```python
from build123d import *
from build123d.topology import SkipClean

# Parameters (mm, degrees)
SKETCH_1_R               = 22.5
EXTRUDE_1_DEPTH          = 13.4
SKETCH_2_R               = 2.1
EXTRUDE_2_DEPTH          = 4
FILLET_1_R               = 3.69
EXTRUDE_3_DEPTH          = 9.5
EXTRUDE_5_DEPTH          = 2
EXTRUDE_4_DEPTH          = 4.5
CUT_EXTRUDE_START        = -11
SKETCH_5_R               = 21.001588026
CUT_EXTRUDE_1_DEPTH      = 11
SKETCH_6_R               = 8
CUT_EXTRUDE_2_DEPTH      = 3
PATTERN_CIRCULAR_1_COUNT = 3
EXTRUDE_START            = -9
EXTRUDE_6_DEPTH          = 9
EXTRUDE_7_DEPTH          = 1
EXTRUDE_8_DEPTH          = 7
CHAMFER_1_SIZE           = 0.5
SKETCH_13_R              = 9.5
CUT_EXTRUDE_4_DEPTH      = 2
EXTRUDE_10_DEPTH         = 13.4


with BuildPart() as part:
    # Эскиз1 → Бобышка-Вытянуть1 (new body)
    with BuildSketch(Plane(origin=(0, 0, 0), x_dir=(1, 0, 0), z_dir=(0, 1, 0))):
        with Locations(Location((0, 0, 0), (0, 0, 270))):
            Circle(SKETCH_1_R)
    extrude(amount=EXTRUDE_1_DEPTH)

    # Эскиз2 → Бобышка-Вытянуть2 (add)
    # profile 1 of 2: a face of its own
    with BuildSketch(Plane.XZ):
        with BuildLine():
            Line((22.193692798, 3.7), (32.5, 3.7))
            Line((32.5, 3.7), (32.5, -3.7))
            Line((32.5, -3.7), (22.193692798, -3.7))
            ThreePointArc((22.193692798, -3.7), (22.5, 0), (22.193692798, 3.7))
        make_face()
        with Locations(Location((28.5, 0, 0), (0, 0, 270))):
            Circle(SKETCH_2_R, mode=Mode.SUBTRACT)
    # profile 2 of 2: a face of its own
    with BuildSketch(Plane.XZ):
        with BuildLine():
            Line((-22.193692798, -3.7), (-32.5, -3.7))
            Line((-32.5, -3.7), (-32.5, 3.7))
            Line((-32.5, 3.7), (-22.193692798, 3.7))
            ThreePointArc((-22.193692798, 3.7), (-22.5, 0), (-22.193692798, -3.7))
        make_face()
        with Locations(Location((-28.5, 0, 0), (0, 0, 90))):
            Circle(SKETCH_2_R, mode=Mode.SUBTRACT)
    extrude(amount=-EXTRUDE_2_DEPTH)

    # Скругление1
    fillet_1_edges = [part.edges().sort_by_distance(p)[0] for p in [
        (-32.5, 2, -3.7),
        (-32.5, 2, 3.7),
        (32.5, 2, 3.7),
        (32.5, 2, -3.7),
    ]]
    fillet(fillet_1_edges, radius=FILLET_1_R)

    # Эскиз3 → Бобышка-Вытянуть3 (add)
    with BuildSketch(Plane(origin=(0, 13.4, 0), x_dir=(1, 0, 0), z_dir=(0, 1, 0))):
        with BuildLine():
            Line((-1, 22.477766793), (-1, 20.977766793))
            ThreePointArc((-1, 20.977766793), (0, 21.001588026), (1, 20.977766793))
            Line((1, 20.977766793), (1, 22.477766793))
            ThreePointArc((1, 22.477766793), (0, 22.5), (-1, 22.477766793))
        make_face()
        with BuildLine():
            Line((19.966317063, -10.372857993), (18.667278957, -9.622857993))
            ThreePointArc((18.667278957, -9.622857993), (18.18790875, -10.500794013), (17.667278957, -11.3549088))
            Line((17.667278957, -11.3549088), (18.966317063, -12.1049088))
            ThreePointArc((18.966317063, -12.1049088), (19.485571585, -11.25), (19.966317063, -10.372857993))
        make_face()
        with BuildLine():
            Line((-18.966317063, -12.1049088), (-17.667278957, -11.3549088))
            ThreePointArc((-17.667278957, -11.3549088), (-18.18790875, -10.500794013), (-18.667278957, -9.622857993))
            Line((-18.667278957, -9.622857993), (-19.966317063, -10.372857993))
            ThreePointArc((-19.966317063, -10.372857993), (-19.485571585, -11.25), (-18.966317063, -12.1049088))
        make_face()
    extrude(amount=EXTRUDE_3_DEPTH)

    # Эскиз7 → Бобышка-Вытянуть5 (add)
    with BuildSketch(Plane.ZY.offset(1)):
        Polygon((-22.477766793, 22.9), (-23.477766793, 21.4), (-22.477766793, 21.4), align=None)
    extrude_5 = extrude(amount=-EXTRUDE_5_DEPTH)

    # Эскиз4 → Бобышка-Вытянуть4 (add)
    with BuildSketch(Plane(origin=(0, 13.4, 0), x_dir=(1, 0, 0), z_dir=(0, 1, 0))):
        with BuildLine():
            Line((-2.5, -20.860679775), (-2.5, -22.360679775))
            ThreePointArc((-2.5, -22.360679775), (0, -22.5), (2.5, -22.360679775))
            Line((2.5, -22.360679775), (2.5, -20.860679775))
            ThreePointArc((2.5, -20.860679775), (0, -21.009949088), (-2.5, -20.860679775))
        make_face()
        with BuildLine():
            Line((-16.815878625, 12.595403397), (-18.114916731, 13.345403397))
            ThreePointArc((-18.114916731, 13.345403397), (-19.485571585, 11.25), (-20.614916731, 9.015276378))
            Line((-20.614916731, 9.015276378), (-19.315878625, 8.265276378))
            ThreePointArc((-19.315878625, 8.265276378), (-18.195149642, 10.504974544), (-16.815878625, 12.595403397))
        make_face()
        with BuildLine():
            Line((19.315878625, 8.265276378), (20.614916731, 9.015276378))
            ThreePointArc((20.614916731, 9.015276378), (19.485571585, 11.25), (18.114916731, 13.345403397))
            Line((18.114916731, 13.345403397), (16.815878625, 12.595403397))
            ThreePointArc((16.815878625, 12.595403397), (18.195149642, 10.504974544), (19.315878625, 8.265276378))
        make_face()
    extrude(amount=EXTRUDE_4_DEPTH)

    # Эскиз5 → Вырез-Вытянуть1 (cut)
    with SkipClean():  # the faces are left unmerged after this step: merging them gives an invalid solid
        with BuildSketch(Plane(origin=(0, 13.4, 0), x_dir=(1, 0, 0), z_dir=(0, 1, 0)).offset(CUT_EXTRUDE_START)):
            with Locations(Location((0, 0, 0), (0, 0, 87.270803902))):
                Circle(SKETCH_5_R)
        extrude(amount=CUT_EXTRUDE_1_DEPTH, mode=Mode.SUBTRACT)

    # Эскиз6 → Вырез-Вытянуть2 (cut)
    with SkipClean():  # the faces are left unmerged after this step: merging them gives an invalid solid
        with BuildSketch(Plane(origin=(0, 0, 0), x_dir=(-1, 0, 0), z_dir=(0, -1, 0))):
            with Locations(Location((0, 0, 0), (0, 0, 90))):
                Circle(SKETCH_6_R)
        extrude(amount=-CUT_EXTRUDE_2_DEPTH, mode=Mode.SUBTRACT)

    # Круговой массив1: Бобышка-Вытянуть5 ×3 about axis
    with SkipClean():  # the faces are left unmerged after this step: merging them gives an invalid solid
        pattern_circular_1_axis = Axis((0, 0, 0), (0, 1, 0))
        for i in range(1, PATTERN_CIRCULAR_1_COUNT):
            add(extrude_5.rotate(pattern_circular_1_axis, i * 360 / PATTERN_CIRCULAR_1_COUNT))

    # Эскиз8 → Бобышка-Вытянуть6 (add)
    with SkipClean():  # the faces are left unmerged after this step: merging them gives an invalid solid
        with BuildSketch(Plane(origin=(0, 13.4, 0), x_dir=(1, 0, 0), z_dir=(0, 1, 0)).offset(EXTRUDE_START)):
            with BuildLine():
                Line((7.917321695, 23.713203436), (6.638578465, 21.498355192))
                ThreePointArc((6.638578465, 21.498355192), (11.25, 19.485571585), (15.298832503, 16.498355192))
                Line((15.298832503, 16.498355192), (16.577575733, 18.713203436))
                ThreePointArc((16.577575733, 18.713203436), (12.5, 21.650635095), (7.917321695, 23.713203436))
            make_face()
            with BuildLine():
                Line((-7.917321695, -23.713203436), (-6.638578465, -21.498355192))
                ThreePointArc((-6.638578465, -21.498355192), (-11.25, -19.485571585), (-15.298832503, -16.498355192))
                Line((-15.298832503, -16.498355192), (-16.577575733, -18.713203436))
                ThreePointArc((-16.577575733, -18.713203436), (-12.5, -21.650635095), (-7.917321695, -23.713203436))
            make_face()
        extrude(amount=EXTRUDE_6_DEPTH)

    # Эскиз9 → Бобышка-Вытянуть7 (add)
    with SkipClean():  # the faces are left unmerged after this step: merging them gives an invalid solid
        with BuildSketch(Plane(origin=(0, 13.4, 0), x_dir=(1, 0, 0), z_dir=(0, 1, 0))):
            Polygon((8.069392034, 22.476596989), (7.869392034, 22.130186827), (15.230607966, 17.880186827), (15.430607966, 18.226596989), align=None)
            Polygon((-8.069392034, -22.476596989), (-15.430607966, -18.226596989), (-15.230607966, -17.880186827), (-7.869392034, -22.130186827), align=None)
        extrude(amount=EXTRUDE_7_DEPTH)

    # Эскиз10 → Бобышка-Вытянуть8 (add)
    with SkipClean():  # the faces are left unmerged after this step: merging them gives an invalid solid
        with BuildSketch(Plane(origin=(0, 14.4, 0), x_dir=(1, 0, 0), z_dir=(0, 1, 0))):
            Polygon((10.580865705, 21.026596989), (10.380865705, 20.680186827), (12.719134295, 19.330186827), (12.919134295, 19.676596989), align=None)
            Polygon((-10.580865705, -21.026596989), (-12.919134295, -19.676596989), (-12.719134295, -19.330186827), (-10.380865705, -20.680186827), align=None)
        extrude(amount=EXTRUDE_8_DEPTH)

    # Фаска1
    chamfer_1_edges = [part.edges().sort_by_distance(p)[0] for p in [
        (10.480865705, 21.4, -20.853391908),
        (12.819134295, 21.4, -19.503391908),
        (-10.480865705, 21.4, 20.853391908),
        (-12.819134295, 21.4, 19.503391908),
    ]]
    chamfer(chamfer_1_edges, length=CHAMFER_1_SIZE)

    # Эскиз11 → Повернуть1 (revolve)
    with SkipClean():  # the faces are left unmerged after this step: merging them gives an invalid solid
        with BuildSketch(Plane(origin=(0, 0, 0), x_dir=(0, 0, -1), z_dir=(1, 0, 0))):
            Polygon((20.5, 2.4), (17.5, 2.4), (4.99, 9.622651868), (4.99, 10.9), (15.74, 10.9), (15.74, 11.4), (-0.01, 11.4), (-0.01, 10.9), (4.49, 10.9), (4.49, 9.333976733), (17.366025404, 1.9), (20.5, 1.9), align=None)
        revolve(axis=Axis((0, 0, 0.01), (0, 1, 0)))

    # Эскиз13 → Вырез-Вытянуть4 (cut)
    with SkipClean():  # the faces are left unmerged after this step: merging them gives an invalid solid
        with BuildSketch(Plane.XZ):
            with Locations(Location((0, 0, 0), (0, 0, 270))):
                Circle(SKETCH_13_R)
        extrude(amount=-CUT_EXTRUDE_4_DEPTH, mode=Mode.SUBTRACT)

    # Эскиз15 → Бобышка-Вытянуть10 (add)
    with SkipClean():  # the faces are left unmerged after this step: merging them gives an invalid solid
        with BuildSketch(Plane.XZ):
            with BuildLine():
                Line((-21.937410968, 5), (-22.75, 5))
                Line((-22.75, 5), (-22.75, -5))
                Line((-22.75, -5), (-21.937410968, -5))
                ThreePointArc((-21.937410968, -5), (-22.5, 0), (-21.937410968, 5))
            make_face()
            with BuildLine():
                Line((22.75, 5), (22.75, -5))
                Line((22.75, -5), (21.937410968, -5))
                ThreePointArc((21.937410968, -5), (22.5, 0), (21.937410968, 5))
                Line((21.937410968, 5), (22.75, 5))
            make_face()
        extrude(amount=-EXTRUDE_10_DEPTH)


solid = part.part
```
Could you check a few things on this model? Use its own coordinates, in mm. A direction names the side the tool comes from. Round coordinates to 2 decimals unless told otherwise and drop trailing zeros. Order: outer loops, then holes, each group sorted by start corner. A loop starts at its lowest first (then second) coordinate and runs counter-clockwise, first axis right, second up. Notation, with made-up numbers: M 78,-31.5 L 107,-31.5 A21 ccw 107,-9.5 Z; hole C 55.25,29 d1. An arc over 180 degrees is marked long. One line per question, with ' | ' between items. Start each with the question number.
(1) For faces 4 (the face through (5.474, 9.272, 1.226)), 5 (the face through (15.93, 8.84, -17.59)), 6 (the face through (-15.616, 11.154, 2.06)), 7 (the face through (2.5, 16, 22)), 8 (the face through (-7.81, 2.2, 1.73)), which set-ups out of +Z, -Z, +X, -X, +Y, -Y let a thin tool reach every point of the face, with its end or its side?
(2) Thinking about a two-plate mould opening in Z: for faces 1 (the face through (-19.886, 22.16, 11.498)), 2 (the face through (1, 18, -22)), 3 (the face through (-26.637, 1.972, 0.969)), which applies, +Z half, -Z half, draft (parallel to the pull), parting line (faces both ways), or undercut?
(3) Suppose I cut it at B-B on y = 15.75. Count the separate pieces of the cut face and the enclosed holes in it, then the cut area to 3 significant figures.
(4) Suppose I cut it at A-A on y = 7.25. List the corners of the cut face in (x, z) for me.
(5) Suppose I cut it at C-C on y = 12.5. List the corners of the cut face in (x, z) for me.
(6) Please list where these lines run through material, in increasing order: line 1 along Y through (x, z) = (-4, -12.5); line 2 along X through (y, z) = (7, 0); line 3 along Z through (x, y) = (0, 6.5).
(7) For P1, Ø8, axis at y = 3.5, z = 13.5, coming from the +X side; P2, Ø12, axis at y = 11.5, z = -15, coming from the -X side; P3, Ø1.4, axis at x = -14.5, z = 19, coming from the +Y side, each with a flat end and sliding along its axis, tell me the tip position at first contact or that it passes through.
Geometry results:
1) face 4: none | face 5: +X, +Y, -Y | face 6: +Y | face 7: +Z, -Z, +X, +Y | face 8: -Y
2) face 1: +Z half | face 2: draft | face 3: undercut
3) separate pieces: 8 | enclosed holes: 0 | area: 33.6 mm²
4) outline: M -22.75,-5 L -21.94,-5 A22.5 ccw 6.64,-21.5 L 7.92,-23.71 A25 ccw 16.58,-18.71 L 15.3,-16.5 A22.5 ccw 21.94,-5 L 22.75,-5 L 22.75,5 L 21.94,5 A22.5 ccw -6.64,21.5 L -7.92,23.71 A25 ccw -16.58,18.71 L -15.3,16.5 A22.5 ccw -21.94,5 L -22.75,5 Z; C 0,0.01 d18.22; hole C 0,0 d42; hole C 0,0.01 d16.22
5) outline: M -22.75,-5 L -21.94,-5 A22.5 ccw 6.64,-21.5 L 7.92,-23.71 A25 ccw 16.58,-18.71 L 15.3,-16.5 A22.5 ccw 21.94,-5 L 22.75,-5 L 22.75,5 L 21.94,5 A22.5 ccw -6.64,21.5 L -7.92,23.71 A25 ccw -16.58,18.71 L -15.3,16.5 A22.5 ccw -21.94,5 L -22.75,5 Z; hole C 0,0 d42
6) line 1: 0 to 2.4, 4.35 to 4.93, 10.9 to 11.4 | line 2: -22.75 to -21, -9.54 to -8.54, 8.54 to 9.54, 21 to 22.75 | line 3: -22.5 to -21, -10.4 to -9.4, 9.42 to 10.42, 21 to 22.5
7) P1: x = 20.4 | P2: x = -20.62 | P3: y = 14.4
